The model under review builds one solid part; all positions refer to its coordinate system, in mm. Face numbers are marked on the shaded views. Round coordinates to 2 decimals unless told otherwise and drop trailing zeros. Loops run counter-clockwise (first coordinate to the right, second up) from the corner with the lowest first, then second, coordinate; pieces in that order, holes last. Notation, with made-up numbers: (77.5, 42.5) -> (133.5, 42.5) arc R17 ccw to (133.5, 59.5) -> close; hole circle Ø9 at (-27.5, 59.5). An arc over 180 degrees is marked (long way). Return JSON: item names as keys, results as strings. Group by question number.
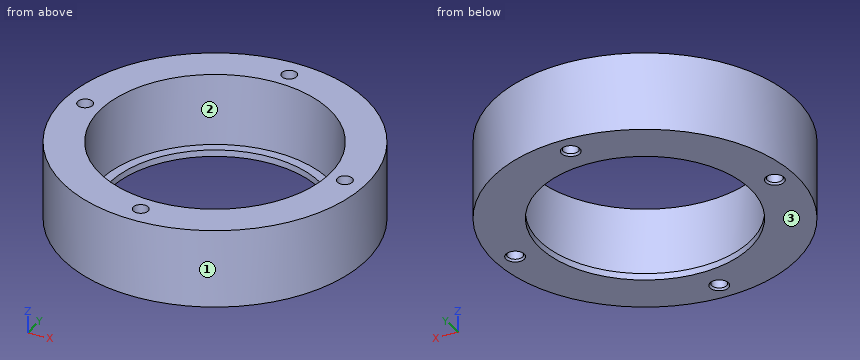
```python
from build123d import *

# Parameters (mm, degrees)
SKETCH1_R           = 34.5
SKETCH1_R_2         = 24
BOSS_EXTRUDE1_DEPTH = 1.5
SKETCH3_R           = 34.5
SKETCH3_R_2         = 26.15
BOSS_EXTRUDE2_DEPTH = 16.4
SKETCH4_R           = 1.7
CUT_EXTRUDE1_DEPTH  = 52.970279968
CHAMFER1_SIZE       = 0.4


with BuildPart() as part:
    # Sketch1 → Boss-Extrude1 (new body)
    with BuildSketch(Plane.XY):
        Circle(SKETCH1_R)
        Circle(SKETCH1_R_2, mode=Mode.SUBTRACT)
    extrude(amount=BOSS_EXTRUDE1_DEPTH)

    # Sketch3 → Boss-Extrude2 (add)
    with BuildSketch(Plane.XY.offset(1.5)):
        Circle(SKETCH3_R)
        Circle(SKETCH3_R_2, mode=Mode.SUBTRACT)
    extrude(amount=BOSS_EXTRUDE2_DEPTH)

    # Sketch4 → Cut-Extrude1 (cut, through all)
    with BuildSketch(Plane.XY.offset(17.9)):
        with Locations((0, 30)):
            Circle(SKETCH4_R)
        with Locations((30, 0)):
            Circle(SKETCH4_R)
        with Locations((0, -30)):
            Circle(SKETCH4_R)
        with Locations((-30, 0)):
            Circle(SKETCH4_R)
    extrude(amount=-CUT_EXTRUDE1_DEPTH, mode=Mode.SUBTRACT)

    # Chamfer1
    chamfer1_edges = [part.edges().sort_by_distance(p)[0] for p in [
        (-1.7, 30, 0),
        (28.3, 0, 0),
        (-1.7, -30, 0),
        (-31.7, 0, 0),
    ]]
    chamfer(chamfer1_edges, length=CHAMFER1_SIZE)


solid = part.part
```
1. We need section D-D, the plane y = -30. Write out the cut boundary in (x, z), then the cut area to 3 significant figures.
2. For P1, Ø2, axis at x = 0, y = -30, coming from the -Z side; P2, Ø4, axis at y = -15, z = 8, coming from the +X side; P3, Ø2, axis at y = -14, z = 13.5, coming from the -X side; P4, Ø3, axis at x = 5.5, z = 8, coming from the +Y side, all flat-tipped, find the tip position at first contact; note any pin that passes through.
3. We need section A-A, the plane y = 0. Write out the cut boundary in (x, z), then the cut area to 3 significant figures.
4. Draft analysis for pull direction X (two halves, no side actions). For the marked faces 1, 2 and 3, state which applies: pulls with the +X half, pulls with the -X half, needs draft (parallel to the pull), parting line crosses it, or undercut.
5. Wall thickness on line 1 (Y direction, x = 0, z = 9); line 2 (Y direction, x = 1, z = 2); line 3 (X direction, y = -10, z = 10.5): over which ranges is each line inside the solid? List them lowest first.
6. We need section C-C, the plane z = 13.5. Write out the cut boundary in (x, y), then the cut area to 3 significant figures.
Check sheet entries:
{
 "1": {"outline": "(-17.04, 0) -> (-2.1, 0) -> (-1.7, 0.4) -> (-1.7, 17.9) -> (-17.04, 17.9) -> close; (1.7, 0.4) -> (2.1, 0) -> (17.04, 0) -> (17.04, 17.9) -> (1.7, 17.9) -> close", "area": "549 mm²"},
 "2": {"P1": "passes through", "P2": "stops at x = 31.96", "P3": "stops at x = -31.96", "P4": "stops at y = 34.27"},
 "3": {"outline": "(-34.5, 0) -> (-32.1, 0) -> (-31.7, 0.4) -> (-31.7, 17.9) -> (-34.5, 17.9) -> close; (-28.3, 0.4) -> (-27.9, 0) -> (-24, 0) -> (-24, 1.5) -> (-26.15, 1.5) -> (-26.15, 17.9) -> (-28.3, 17.9) -> close; (24, 0) -> (27.9, 0) -> (28.3, 0.4) -> (28.3, 17.9) -> (26.15, 17.9) -> (26.15, 1.5) -> (24, 1.5) -> close; (31.7, 0.4) -> (32.1, 0) -> (34.5, 0) -> (34.5, 17.9) -> (31.7, 17.9) -> close", "area": "183 mm²"},
 "4": {"face 1": "parting line crosses it", "face 2": "undercut", "face 3": "needs draft"},
 "5": {"line 1": "y = -34.5 to -31.7, -28.3 to -26.15, 26.15 to 28.3, 31.7 to 34.5", "line 2": "y = -34.49 to -31.37, -28.63 to -26.13, 26.13 to 28.63, 31.37 to 34.49", "line 3": "x = -33.02 to -24.16, 24.16 to 33.02"},
 "6": {"outline": "circle Ø69 at (0, 0); hole circle Ø3.4 at (-30, 0); hole circle Ø52.3 at (0, 0); hole circle Ø3.4 at (0, -30); hole circle Ø3.4 at (0, 30); hole circle Ø3.4 at (30, 0)", "area": "1,550 mm²"}
}
